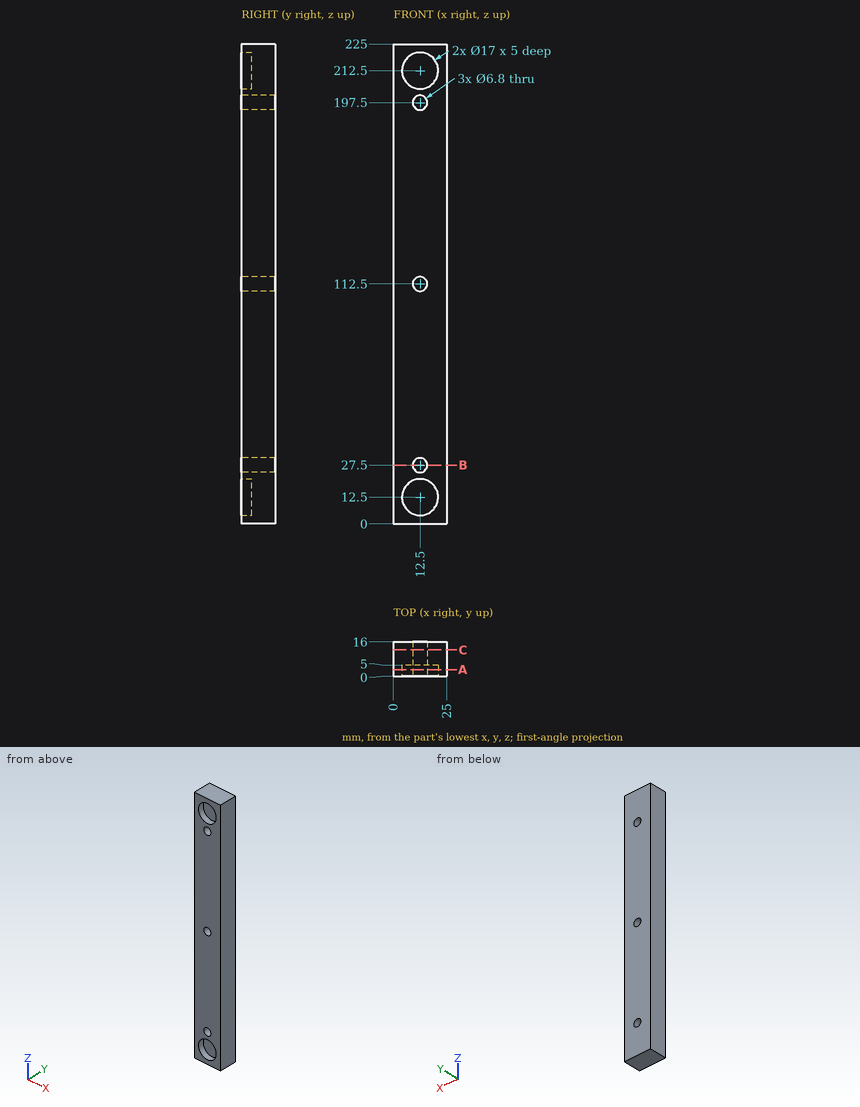
Geometry: see drawing. Coordinates: mm, zero at the bounding-box minimum. Round coordinates to 2 decimals unless told otherwise and drop trailing zeros. Loops run counter-clockwise (first coordinate to the right, second up) from the corner with the lowest first, then second, coordinate; pieces in that order, holes last. Notation, with made-up numbers: (56, 75.5) -> (60, 75.5) arc R28 ccw to (60, 109.5) -> close; hole circle Ø8 at (32.25, 23.5). An arc over 180 degrees is marked (long way). Write each question's results on one line, items separated by ' | '.
Item 1: Cut plane C-C on y = 12.25. Return the cut outline in (x, z).
Answers below:
outline: (0, 0) -> (25, 0) -> (25, 225) -> (0, 225) -> close; hole circle Ø6.8 at (12.5, 27.5); hole circle Ø6.8 at (12.5, 112.5); hole circle Ø6.8 at (12.5, 197.5)
Item 2: Line query: probe 1 along Z at (x, y) = (12, 12); probe 2 along X at (y, z) = (3.5, 112.5); probe 3 along Z at (x, y) = (10.5, 11.5). Output: solid intervals per line, ascending. Write a range as [from, to].
Answers below:
probe 1: z = [0, 24.14], [30.86, 109.14], [115.86, 194.14], [200.86, 225] | probe 2: x = [0, 9.1], [15.9, 25] | probe 3: z = [0, 24.75], [30.25, 109.75], [115.25, 194.75], [200.25, 225]
Item 3: Cut plane B-B on z = 27.5. Return the cut outline in (x, y), and give its area (3 significant figures).
Answers below:
outline: (0, 0) -> (9.1, 0) -> (9.1, 16) -> (0, 16) -> close; (15.9, 0) -> (25, 0) -> (25, 16) -> (15.9, 16) -> close | area: 291 mm²
Item 4: Cut plane A-A on y = 3. Return the cut outline in (x, z), and give its area (3 significant figures).
Answers below:
outline: (0, 0) -> (25, 0) -> (25, 225) -> (0, 225) -> close; hole circle Ø17 at (12.5, 12.5); hole circle Ø17 at (12.5, 212.5); hole circle Ø6.8 at (12.5, 27.5); hole circle Ø6.8 at (12.5, 112.5); hole circle Ø6.8 at (12.5, 197.5) | area: 5,060 mm²
